Read the model definition and answer for the solid it produces. Units are mm, in the model's axes. Face numbers are marked on the shaded views. A direction names the side the tool comes from. Coordinates: 2 decimals unless noted, no trailing zeros. Write each loop counter-clockwise with the first axis right and the second up, starting at its lowest first coordinate (ties: lowest second). Pieces come first, ordered by that corner, then holes.
(1) The part is cut by section B-B, the plane y = 7.25. Determine the outline of the cut face in (x, z).
(2) Straight lines are drawn through the part: line 1 along X through (y, z) = (0.45, 0); line 2 along Z through (x, y) = (15, 3.5); line 3 along Z through (x, y) = (17, 12.5). For each, find the intervals that lie inside material, in ascending order.
(3) Which of the six approach directions +Z, -Z, +X, -X, +Y, -Y give full straight-line access (tool end or side, diameter ignored) to the marked faces 1 and 2?
(4) The part is cut by section D-D, the plane x = 22. Determine the outline of the cut face in (y, z), and give its area (3 significant figures).
(5) Determine the mould class of the marked faces 3, 4 and 5 for opening direction Z: pulls with the +Z half, pulls with the -Z half, needs draft (parallel to the pull), parting line crosses it, or undercut.
(6) The part is cut by section C-C, the plane z = -59.5. Determine the outline of the cut face in (x, y).
(7) The part is cut by section A-A, the plane x = 0. Determine the outline of the cut face in (y, z).
(8) Given pin 1 (4 mm diameter, centred on x = 52.5, y = 12.5, fed in from -Z); pin 2 (3 mm diameter, centred on y = 12, z = 51.5, fed in from -X); pin 3 (6 mm diameter, centred on y = 12.5, z = 10.5, fed in from +X); pin 4 (24 mm diameter, centred on x = 3.5, z = 5, fed in from +Y), each flat-ended and moving along its own axis, determine where each tip first touches the part or whether it passes through.
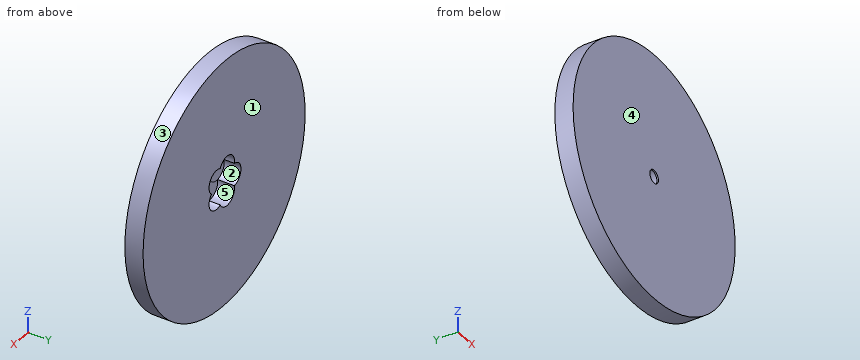
```python
from build123d import *

# Parameters (mm, degrees)
SKETCH1_R           = 95
BOSS_EXTRUDE1_DEPTH = 14
SKETCH2_R           = 5
CUT_EXTRUDE1_DEPTH  = 136.077755386
SKETCH3_R           = 8.797146217
CUT_EXTRUDE2_DEPTH  = 12.856004
CIRPATTERN1_START   = 1.143995707
CIRPATTERN1_DEPTH   = 12.856004293


# Read off the part's stored shape, not the designer's step: CirPattern1
with BuildPart() as part:
    # Sketch1 → Boss-Extrude1 (new body)
    with BuildSketch(Plane(origin=(0, 0, 0), x_dir=(1, 0, 0), z_dir=(0, 1, 0))):
        with Locations(Location((0, 0, 0), (0, 0, 270))):
            Circle(SKETCH1_R)
    extrude(amount=BOSS_EXTRUDE1_DEPTH)

    # Sketch2 → Cut-Extrude1 (cut, through all)
    with BuildSketch(Plane(origin=(0, 0, 0), x_dir=(1, 0, 0), z_dir=(0, 1, 0))):
        with Locations(Location((0, 0, 0), (0, 0, 270))):
            Circle(SKETCH2_R)
    extrude(amount=CUT_EXTRUDE1_DEPTH, mode=Mode.SUBTRACT)

    # Sketch3 → Cut-Extrude2 (cut)
    with BuildSketch(Plane(origin=(0, 14, 0), x_dir=(1, 0, 0), z_dir=(0, 1, 0))):
        with Locations((-10.953492751, 0)):
            Circle(SKETCH3_R)
    extrude(amount=-CUT_EXTRUDE2_DEPTH, mode=Mode.SUBTRACT)

    # CirPattern1 outline → CirPattern1 (cut)
    with BuildSketch(Plane(origin=(0, 0, 0), x_dir=(1, 0, 0), z_dir=(0, 1, 0)).offset(CIRPATTERN1_START)):
        with BuildLine():
            ThreePointArc((-3.085281719, -3.93459486), (-6.791330571, -7.750237902), (-12.019078058, -8.732371357))
            ThreePointArc((-12.019078058, -8.732371357), (-6.10328309, -18.783973891), (4.590879305, -14.129273657))
            ThreePointArc((4.590879305, -14.129273657), (15.978602575, -11.609134309), (14.856397507, 0))
            ThreePointArc((14.856397507, 0), (15.978602575, 11.609134309), (4.590879305, 14.129273657))
            ThreePointArc((4.590879305, 14.129273657), (-6.10328309, 18.783973891), (-12.019078058, 8.732371357))
            ThreePointArc((-12.019078058, 8.732371357), (-6.791330571, 7.750237902), (-3.085281719, 3.93459486))
            ThreePointArc((-3.085281719, 3.93459486), (5, 0), (-3.085281719, -3.93459486))
        make_face()
    extrude(amount=CIRPATTERN1_DEPTH, mode=Mode.SUBTRACT)


solid = part.part
```
Computed:
1. outline: circle Ø190 at (0, 0); hole (-12.02, -8.73) arc R8.8 ccw to (4.59, -14.13) arc R8.8 ccw to (14.86, 0) arc R8.8 ccw to (4.59, 14.13) arc R8.8 ccw to (-12.02, 8.73) arc R8.8 ccw to start
2. line 1: x = -95 to -5, 5 to 95
2. line 2: z = -93.81 to -12.74, -0.14 to 0.14, 12.74 to 93.81
2. line 3: z = -93.47 to -9.78, -3.1 to 3.1, 9.78 to 93.47
3. face 1: +Z, -Z, +X, -X, +Y
3. face 2: +Y
4. outline: (0, -92.42) - (14, -92.42) - (14, 92.42) - (0, 92.42) - close
4. area: 2,590 mm2
5. face 3: parting line crosses it
5. face 4: needs draft
5. face 5: undercut
6. outline: (-74.06, 0) - (74.06, 0) - (74.06, 14) - (-74.06, 14) - close
7. outline: (0, -95) - (14, -95) - (14, -18.54) - (1.14, -18.54) - (1.14, -5) - (0, -5) - close; (0, 5) - (1.14, 5) - (1.14, 18.54) - (14, 18.54) - (14, 95) - (0, 95) - close
8. pin 1: stops at z = -80.47
8. pin 2: stops at x = -80.78
8. pin 3: stops at x = 94.7
8. pin 4: stops at y = 14
